Check sheet for the modelled part. Datum: model origin and axes. Units: mm. Face numbers are marked on the shaded views. A direction names the side the tool comes from. Give positions to 0.01 mm unless a question says otherwise; leave off trailing zeros. Order: outer loops, then holes, each group sorted by start corner. A loop starts at its lowest first (then second) coordinate and runs counter-clockwise, first axis right, second up.
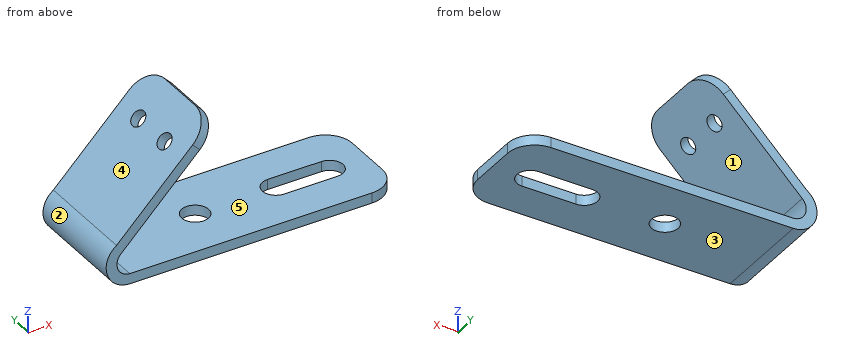
from build123d import *

# Parameters (mm, degrees)
F0_W     = 50
F0_H     = 19.05
F0_R     = 2.5
F1_DEPTH = 1.9
F2_R     = 5
F4_DEPTH = 19.05
F5_R     = 5
F6_R     = 1.5
F7_DEPTH = 5


with BuildPart() as f1:
    # F0 (on Top) → F1 (new body)
    with BuildSketch(Plane.XY):
        with Locations((7, 0)):
            Rectangle(F0_W, F0_H)
        Circle(F0_R, mode=Mode.SUBTRACT)
        with BuildLine():
            ThreePointArc((25.0017541021, 2.4929631711), (26.7634116596, 1.762171322), (27.4929637882, 0))
            ThreePointArc((27.4929637882, 0), (26.7634116596, -1.762171322), (25.0017541021, -2.4929631711))
            Line((25.0017541021, -2.4929631711), (15.0017590529, -2.4999993811))
            ThreePointArc((15.0017590529, -2.4999993811), (12.5, 0), (15.0017590529, 2.4999993811))
            Line((15.0017590529, 2.4999993811), (25.0017541021, 2.4929631711))
        make_face(mode=Mode.SUBTRACT)
    extrude(amount=F1_DEPTH)

    # F2
    f2_edges = [f1.edges().sort_by_distance(p)[0] for p in [
        (32, -9.525, 0.95),
        (32, 9.525, 0.95),
    ]]
    fillet(f2_edges, radius=F2_R)

    # F3 (on face) → F4 (join)
    with BuildSketch(Plane.XZ.offset(9.525)):
        with BuildLine():
            Line((-2.7983656003, 25.7148731307), (-20.47603513, 8.037203601))
            ThreePointArc((-20.47603513, 8.037203601), (-22.2049789443, 3.1045649079), (-18, 0))
            Line((-18, 0), (-18, 1.9))
            ThreePointArc((-18, 1.9), (-20.2226399871, 3.4906627434), (-19.6607572738, 6.1654756887))
            Line((-19.6607572738, 6.1654756887), (-1.454862716, 24.3713702464))
            Line((-1.454862716, 24.3713702464), (-2.7983656003, 25.7148731307))
        make_face()
    extrude(amount=-F4_DEPTH)

    # F5
    f5_edges = [f1.edges().sort_by_distance(p)[0] for p in [
        (-2.126614, -9.525, 25.043122),
        (-2.126614, 9.525, 25.043122),
    ]]
    fillet(f5_edges, radius=F5_R)

    # F6 (on face) → F7 (cut)
    with BuildSketch(Plane(origin=(-14.2566193655, 0, 14.2566193655), x_dir=(0, -1, 0), z_dir=(-0.7071067812, 0, 0.7071067812))):
        with Locations((-3.9354462066, 8.6580958872)):
            Circle(F6_R)
        with Locations((3.9404836009, 8.701013138)):
            Circle(F6_R)
    extrude(amount=-F7_DEPTH, mode=Mode.SUBTRACT)


solid = f1.part
1) Section check B-B, the plane y = 0. Record the cut outline in (x, z).
Recorded:
outline: (-20.48, 8.04) arc R4.4 ccw to (-18, 0) - (-2.5, 0) - (-2.5, 1.9) - (-18, 1.9) arc R2.5 cw to (-19.66, 6.17) - (-1.45, 24.37) - (-2.8, 25.71) - close; (2.5, 0) - (12.5, 0) - (12.5, 1.9) - (2.5, 1.9) - close; (27.49, 0) - (32, 0) - (32, 1.9) - (27.49, 1.9) - close
2) Section check A-A, the plane x = 0. Record the cut outline in (y, z) (3 decimals), then the cut area to 3 significant figures.
Recorded:
outline: (-9.525, 0) - (-2.5, 0) - (-2.5, 1.9) - (-9.525, 1.9) - close; (2.5, 0) - (9.525, 0) - (9.525, 1.9) - (2.5, 1.9) - close
area: 26.7 mm2
3) Depth check by flat-ended pin: pin 1 Ø1.5 at (x, y) = (26, -2.5) entering from -Z; pin 2 Ø2 at (y, z) = (-4.5, 17) entering from +X; pin 3 Ø3 at (x, y) = (-6, -3.5) entering from +Z; pin 4 Ø8 at (x, z) = (-0.5, 17.5) entering from -Y. Enter the tip coordinate at first touch or a pass-through.
Recorded:
pin 1: stops at z = 0
pin 2: stops at x = -7.83
pin 3: stops at z = 24.01
pin 4: passes through
4) Draft check along Z on the marked faces 3, 4 and 5. Enter one of: +Z half, -Z half, draft (parallel to the pull), parting line (faces both ways), or undercut.
Recorded:
face 3: -Z half
face 4: +Z half
face 5: undercut
5) Material ranges on L1, parallel to Y at x = 0, z = 1.4 (3 decimals); L2, parallel to Z at x = 13, y = -3.5; L3, parallel to Z at x = -11.5, y = 4.5, recorded low to high.
Recorded:
L1: y = -9.525 to -2.5, 2.5 to 9.525
L2: z = 0 to 1.9
L3: z = 0 to 1.9, 14.33 to 17.01
6) Section check C-C, the plane y = 3.25. Record the cut outline in (x, z), then the cut area to 3 significant figures.
Recorded:
outline: (-20.48, 8.04) arc R4.4 ccw to (-18, 0) - (32, 0) - (32, 1.9) - (-18, 1.9) arc R2.5 cw to (-19.66, 6.17) - (-7.73, 18.09) - (-9.08, 19.44) - close; (-7.19, 21.32) - (-5.85, 19.98) - (-1.45, 24.37) - (-2.8, 25.71) - close
area: 155 mm2
7) Section check D-D, the plane x = -14. Record the cut outline in (y, z) (3 decimals).
Recorded:
outline: (-9.525, 0) - (9.525, 0) - (9.525, 1.9) - (-9.525, 1.9) - close; (-9.525, 11.826) - (9.525, 11.826) - (9.525, 14.513) - (-9.525, 14.513) - close
8) Set-up check for the marked faces 1 and 2: record each of +Z, -Z, +X, -X, +Y, -Y from which the full face is reachable in a straight line by a thin tool's end or side.
Recorded:
face 1: +X, +Y, -Y
face 2: -X, +Y, -Y
